For this review, use the dimensioned drawing (mm, ordinates from the lowest corner) and the shaded views. A direction names the side the tool comes from. Coordinates: 2 decimals unless noted, no trailing zeros. Write each loop counter-clockwise with the first axis right and the second up, starting at its lowest first coordinate (ties: lowest second). Pieces come first, ordered by that corner, then holes.
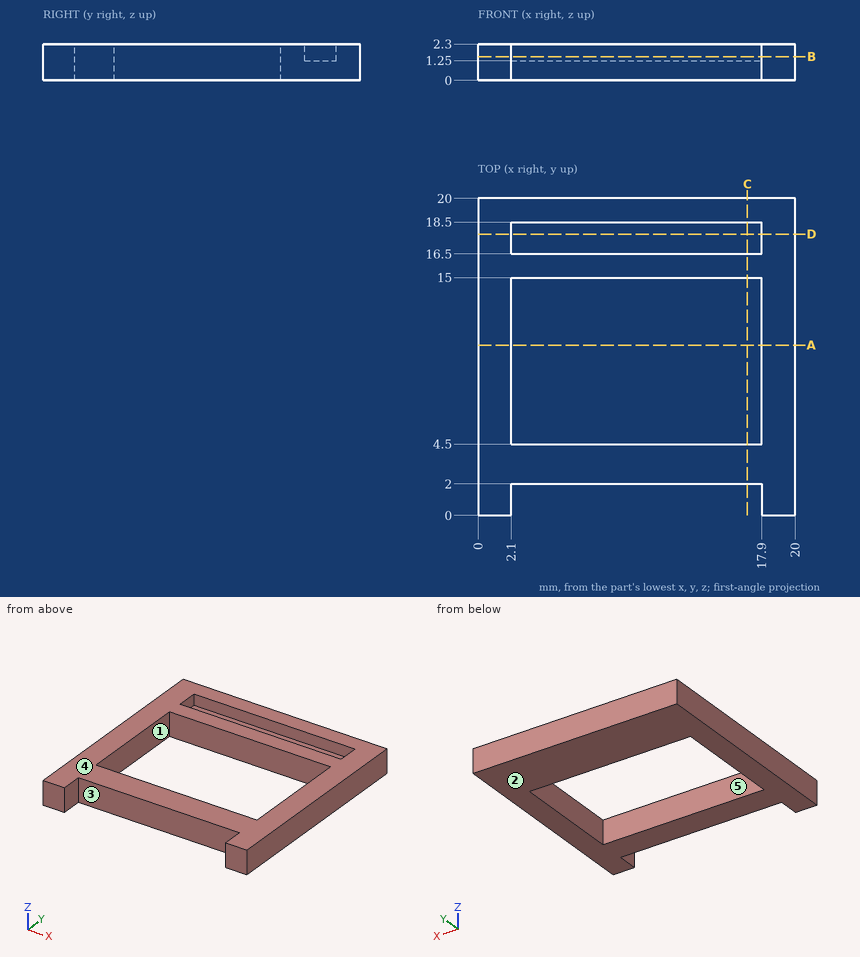
Item 1: Take a section at A-A, the plane y = 10.75. Write out the cut boundary in (x, z), plus the area to 3 significant figures.
Solved:
outline: (0, 0) - (2.1, 0) - (2.1, 2.3) - (0, 2.3) - close; (17.9, 0) - (20, 0) - (20, 2.3) - (17.9, 2.3) - close
area: 9.66 mm2
Item 2: Take a section at C-C, the plane x = 17. Write out the cut boundary in (y, z), plus the area to 4 significant figures.
Solved:
outline: (2, 0) - (4.5, 0) - (4.5, 2.3) - (2, 2.3) - close; (15, 0) - (20, 0) - (20, 2.3) - (18.5, 2.3) - (18.5, 1.25) - (16.5, 1.25) - (16.5, 2.3) - (15, 2.3) - close
area: 15.15 mm2
Item 3: To check wall thickness, follow line 1 along Y through (x, z) = (13.25, 2.05); line 2 along Y through (x, z) = (10.25, 0.25); line 3 along X through (y, z) = (8.75, 2.2). State the ranges of each line that lie inside material, in increasing order.
Solved:
line 1: y = 2 to 4.5, 15 to 16.5, 18.5 to 20
line 2: y = 2 to 4.5, 15 to 20
line 3: x = 0 to 2.1, 17.9 to 20
Item 4: Mouldability with a two-part tool opening along Y and no side actions: class the marked faces 3, 4 and 5 as pulls with the +Y half, pulls with the -Y half, needs draft (parallel to the pull), parting line crosses it, or undercut.
Solved:
face 3: pulls with the -Y half
face 4: needs draft
face 5: undercut
Item 5: Take a section at D-D, the plane y = 17.75. Write out the cut boundary in (x, z).
Solved:
outline: (0, 0) - (20, 0) - (20, 2.3) - (17.9, 2.3) - (17.9, 1.25) - (2.1, 1.25) - (2.1, 2.3) - (0, 2.3) - close
Item 6: For pin 1 (1.2 mm diameter, centred on y = 7.5, z = 0.5, fed in from -X); pin 2 (0.5 mm diameter, centred on x = 10.5, z = 1.5, fed in from -Y), all flat-tipped, find the tip position at first contact; note any pin that passes through.
Solved:
pin 1: stops at x = 0
pin 2: stops at y = 2
Item 7: Machinability: for the marked faces 1 and 2, which of the approach directions +Z, -Z, +X, -X, +Y, -Y give a long, thin tool a straight path to every point of the face, cutting with its end or side? Answer none if there is none.
Solved:
face 1: +Z, -Z
face 2: -Z, +X, -X, +Y, -Y
Item 8: Take a section at B-B, the plane z = 1.5. Write out the cut boundary in (x, y).
Solved:
outline: (0, 0) - (2.1, 0) - (2.1, 2) - (17.9, 2) - (17.9, 0) - (20, 0) - (20, 20) - (0, 20) - close; hole (2.1, 4.5) - (17.9, 4.5) - (17.9, 15) - (2.1, 15) - close; hole (2.1, 16.5) - (17.9, 16.5) - (17.9, 18.5) - (2.1, 18.5) - close
